Geometry check sheet. Reference: the model listing, model coordinates, mm. A direction names the side the tool comes from. Give positions to 0.01 mm unless a question says otherwise; leave off trailing zeros. Write each loop counter-clockwise with the first axis right and the second up, starting at its lowest first coordinate (ties: lowest second). Pieces come first, ordered by that corner, then holes. Notation, with made-up numbers: (-28, 83.25) - (30, 83.25) arc R30 ccw to (30, 111.25) - close; hole circle Ø2 at (27.5, 75.5). An arc over 180 degrees is marked (long way). Write item = value, one per line. Start each with the question number.
(1) Draft check along Y on faces 4 (the flat face through (-33.014, -75.647, 12.012)), 5 (the flat face through (-33.014, 75.647, 12.012)), 6 (the flat face through (-39, 0, 33.302)). Enter one of: pulls with the +Y half, pulls with the -Y half, needs draft (parallel to the pull), parting line crosses it, or undercut.
(2) Depth check by flat-ended pin: pin 1 Ø5 at (x, z) = (-34, 11) entering from -Y; pin 2 Ø1.5 at (y, z) = (-21.5, 28.5) entering from +X; pin 3 Ø8 at (y, z) = (-44.5, 12) entering from +X. Enter the tip coordinate at first touch or a pass-through.
(3) Access from +Z, -Z, +X, -X, +Y, -Y to the whole of each face (thin tool, end or side, straight path). Record for faces 1 (the cylindrical face through (-51.74, 1.1, 11.92)), 2 (the flat face through (-41, -1, 37.056)), 3 (the cylindrical face through (-42.794, 1.071, 11.745)).
(4) Thickness scan on L1, parallel to Z at x = -42, y = 53; L2, parallel to Z at x = -37.5, y = -51.5; L3, parallel to Z at x = -42, y = -38.5. Record the ranges inside material, lowest first.
(5) Section check A-A, the plane z = 13.5. Enter the section's corners in (x, y), plus the area to 3 significant figures.
```python
from build123d import *

# Parameters (mm, degrees)
F1_ANGLE = 30
F3_ANGLE = 3


with BuildPart() as f1:
    # F0 (on Front) → F1 (revolve, symmetric)
    with BuildSketch(Plane.XZ) as f1_sk:
        with BuildLine():
            Line((-36.445543, 37.056317), (-49.145543, 37.056317))
            ThreePointArc((-49.145543, 37.056317), (-53.635671, 35.196445), (-55.495543, 30.706317))
            Line((-55.495543, 30.706317), (-55.495543, -7.393194))
            ThreePointArc((-55.495543, -7.393194), (-53.635671, -11.883322), (-49.145543, -13.743194))
            Line((-49.145543, -13.743194), (-36.445543, -13.743194))
            ThreePointArc((-36.445543, -13.743194), (-31.955415, -11.883322), (-30.095543, -7.393194))
            Line((-30.095543, -7.393194), (-30.095543, -1.043439))
            Line((-30.095543, -1.043439), (-42.795543, 5.306317))
            Line((-42.795543, 5.306317), (-42.795543, 18.006317))
            Line((-42.795543, 18.006317), (-30.095543, 24.356317))
            Line((-30.095543, 24.356317), (-30.095543, 30.706317))
            ThreePointArc((-30.095543, 30.706317), (-31.955415, 35.196445), (-36.445543, 37.056317))
        make_face()
    revolve(axis=Axis((249.304457, 0, 5.828281), (0, 0, -1)), revolution_arc=F1_ANGLE / 2)
    revolve(f1_sk.sketch, axis=Axis((249.304457, 0, 5.828281), (0, 0, 1)), revolution_arc=F1_ANGLE / 2)

    # F2 (on face) → F3 (revolve)
    with BuildSketch(Plane(origin=(16.700232, -62.326114, 0), x_dir=(0.965926, 0.258819, 0), z_dir=(0.258819, -0.965926, 0))):
        with BuildLine():
            Line((-42.402958, 26.712616), (-42.402958, 30.706317))
            ThreePointArc((-42.402958, 30.706317), (-43.146153, 32.50055), (-44.940386, 33.243746))
            Line((-44.940386, 33.243746), (-57.640386, 33.243746))
            ThreePointArc((-57.640386, 33.243746), (-59.434619, 32.50055), (-60.177815, 30.706317))
            Line((-60.177815, 30.706317), (-60.177815, -7.393194))
            ThreePointArc((-60.177815, -7.393194), (-59.434619, -9.187427), (-57.640386, -9.930623))
            Line((-57.640386, -9.930623), (-44.940386, -9.930623))
            ThreePointArc((-44.940386, -9.930623), (-43.146153, -9.187427), (-42.402958, -7.393194))
            Line((-42.402958, -7.393194), (-42.402958, -3.399778))
            Line((-42.402958, -3.399778), (-55.102958, 2.949978))
            Line((-55.102958, 2.949978), (-55.102958, 20.362616))
            Line((-55.102958, 20.362616), (-42.402958, 26.712616))
        make_face()
    revolve(axis=Axis((249.304457, 0, 17.638403), (0, 0, 1)), revolution_arc=F3_ANGLE)

    # F4 (on face) → F5 (revolve, cut)
    with BuildSketch(Plane(origin=(16.700232, 62.326114, 0), x_dir=(-0.965926, 0.258819, 0), z_dir=(0.258819, 0.965926, 0))):
        with BuildLine():
            Line((60.236317, -7.393194), (60.236317, 30.706317))
            ThreePointArc((60.236317, 30.706317), (59.475986, 32.541917), (57.640386, 33.302248))
            Line((57.640386, 33.302248), (44.940386, 33.302248))
            ThreePointArc((44.940386, 33.302248), (43.104786, 32.541917), (42.344456, 30.706317))
            Line((42.344456, 30.706317), (42.344456, 26.67646))
            Line((42.344456, 26.67646), (55.044456, 20.32646))
            Line((55.044456, 20.32646), (55.044456, 2.986135))
            Line((55.044456, 2.986135), (42.344456, -3.363621))
            Line((42.344456, -3.363621), (42.344456, -7.393194))
            ThreePointArc((42.344456, -7.393194), (43.104786, -9.228794), (44.940386, -9.989125))
            Line((44.940386, -9.989125), (57.640386, -9.989125))
            ThreePointArc((57.640386, -9.989125), (59.475986, -9.228794), (60.236317, -7.393194))
        make_face()
    revolve(axis=Axis((249.304457, 0, 18.53192), (0, 0, 1)), mode=Mode.SUBTRACT)


solid = f1.part
```
Model answer:
q1.face_4 = pulls with the -Y half
q1.face_5 = pulls with the +Y half
q1.face_6 = undercut
q2.pin_1 = -76.57
q2.pin_2 = -29.21
q2.pin_3 = -38.74
q3.face_1 = none
q3.face_2 = +Z, +X, -X, +Y, -Y
q3.face_3 = +X
q4.L1 = -13.74 to -9.99, 33.3 to 37.06
q4.L2 = -13.74 to -9.99, 0.75 to 4.95, 18.36 to 22.56, 33.3 to 37.06
q4.L3 = -13.74 to -9.99, 1.98 to 21.33, 33.3 to 37.06
q5.outline = (-45.11, -78.89) - (-41.48, -77.92) arc R301.05 cw to (-41.48, 77.92) - (-45.11, 78.89) arc R304.8 ccw to start; (-36.47, -76.57) - (-32.84, -75.6) arc R292.1 cw to (-32.84, 75.6) - (-36.47, 76.57) arc R295.85 ccw to start
q5.area = 1,170 mm²
